from build123d import *

# Parameters (mm, degrees)
F0_W          = 80
F0_H          = 7
F0_R          = 2.6
F1_DEPTH      = 11.5
F2_R          = 3
F3_DEPTH      = 5
F4_R          = 3
F5_DEPTH      = 80.001
F6_W          = 4
F6_H          = 3.5
F7_DEPTH      = 39
F7_DEPTH_BACK = 39
F8_SIZE2      = 6.9282032303
F8_SIZE       = 4
F9_SIZE2      = 1.558836
F9_SIZE       = 0.89999
F10_W         = 2
F10_H         = 10.311042398
F11_DEPTH     = 80.001
F12_R         = 3.5
F13_DEPTH     = 1.75
F14_T4_DEPTH  = 17.5408905874
F14_T9_DEPTH  = 17.5408905874
F15_W         = 3
F15_H         = 1.3
F16_DEPTH     = 7.0010001


# Not quite as in the source:
# - a fillet or chamfer that OpenCascade refuses, or shapes differently, is made with other operations: its cross-section is extruded or revolved along the edge and cut away or added
# - a fillet or chamfer is up to 0.001 mm smaller than in the source, because OpenCascade refuses the exact size


with BuildPart() as f1:
    # F0 (on Front) → F1 (new body)
    with BuildSketch(Plane.XZ):
        Rectangle(F0_W, F0_H)
        with Locations((-33, 0)):
            Circle(F0_R, mode=Mode.SUBTRACT)
        with Locations((-22, 0)):
            Circle(F0_R, mode=Mode.SUBTRACT)
        with Locations((-11, 0)):
            Circle(F0_R, mode=Mode.SUBTRACT)
        Circle(F0_R, mode=Mode.SUBTRACT)
        with Locations((11, 0)):
            Circle(F0_R, mode=Mode.SUBTRACT)
        with Locations((22, 0)):
            Circle(F0_R, mode=Mode.SUBTRACT)
        with Locations((33, 0)):
            Circle(F0_R, mode=Mode.SUBTRACT)
    extrude(amount=F1_DEPTH)

    # F2 (on face) → F3 (cut)
    with BuildSketch(Plane(origin=(0, 0, 0), x_dir=(-1, 0, 0), z_dir=(0, 1, 0))):
        Circle(F2_R)
        with Locations((11, 0)):
            Circle(F2_R)
        with Locations((22, 0)):
            Circle(F2_R)
        with Locations((33, 0)):
            Circle(F2_R)
        with Locations((-11, 0)):
            Circle(F2_R)
        with Locations((-22, 0)):
            Circle(F2_R)
        with Locations((-33, 0)):
            Circle(F2_R)
    extrude(amount=-F3_DEPTH, mode=Mode.SUBTRACT)

    # F4 (on face) → F5 (cut, through all)
    with BuildSketch(Plane(origin=(-40, 0, 0), x_dir=(0, -1, 0), z_dir=(-1, 0, 0))):
        Circle(F4_R)
    extrude(amount=-F5_DEPTH, mode=Mode.SUBTRACT)

    # F6 (on Right) → F7 (cut, two sides)
    with BuildSketch(Plane.YZ) as f7_sk:
        with Locations((-3, 0)):
            Rectangle(F6_W, F6_H)
    extrude(amount=-F7_DEPTH, mode=Mode.SUBTRACT)
    extrude(f7_sk.sketch, amount=F7_DEPTH_BACK, mode=Mode.SUBTRACT)

    # F8
    f8_edges = [f1.edges().sort_by_distance(p)[0] for p in [
        (-40, -11.5, 0),
        (40, -11.5, 0),
    ]]
    f8_side = f1.faces().sort_by_distance((39.196943, -11.5, 0))[0]
    chamfer(f8_edges, length=F8_SIZE, length2=F8_SIZE2, reference=f8_side)

    # F9 (size 0.9 and 1.5588457268 in the source; OpenCascade refuses exactly that, so slightly less here)
    f9_edges = [f1.edges().sort_by_distance(p)[0] for p in [
        (0, -11.5, 3.5),
        (0, -11.5, -3.5),
    ]]
    f9_side = f1.faces().sort_by_distance((0, -11.5, 2.776605))[0]
    chamfer(f9_edges, length=F9_SIZE, length2=F9_SIZE2, reference=f9_side)

    # F10 (on face) → F11 (cut, through all)
    with BuildSketch(Plane(origin=(-40, 0, 0), x_dir=(0, -1, 0), z_dir=(-1, 0, 0))):
        Rectangle(F10_W, F10_H)
    extrude(amount=-F11_DEPTH, mode=Mode.SUBTRACT)

    # F12 (on face) → F13 (cut, through all)
    with BuildSketch(Plane(origin=(0, 0, -3.5), x_dir=(1, 0, 0), z_dir=(0, 0, -1))):
        with Locations((0, 1)):
            Circle(F12_R)
    extrude(amount=-F13_DEPTH, mode=Mode.SUBTRACT)

    # F14: fillet of radius 5 on 2 edges, made by hand


with BuildPart() as f14_tool2:
    # F14_s3 → F14_t4 (new body)
    with BuildSketch(Plane.XY.offset(5.6062317314)):
        with BuildLine():
            ThreePointArc((-6.8738635424, -1), (-4.60515051, -1.5443360566), (-2.8304143998, -3.0588235294))
            ThreePointArc((-2.8304143998, -3.0588235294), (-3.3283967912, -2.0824854735), (-3.5, -1))
            Line((-3.5, -1), (-6.8738635424, -1))
        make_face()
    extrude(amount=-F14_T4_DEPTH)

    split(bisect_by=Plane.XY.offset(1.75), keep=Keep.BOTTOM)


with BuildPart() as f1_1:
    add(f1.part)

    # F14_t1: cut F14_tool2
    add(f14_tool2.part, mode=Mode.SUBTRACT)


with BuildPart() as f14_tool7:
    # F14_s8 → F14_t9 (new body)
    with BuildSketch(Plane.XY.offset(-11.9346588561)):
        with BuildLine():
            ThreePointArc((2.8304143998, -3.0588235294), (4.60515051, -1.5443360566), (6.8738635424, -1))
            Line((6.8738635424, -1), (3.5, -1))
            ThreePointArc((3.5, -1), (3.3283967912, -2.0824854735), (2.8304143998, -3.0588235294))
        make_face()
    extrude(amount=F14_T9_DEPTH)

    split(bisect_by=Plane.XY.offset(1.75), keep=Keep.BOTTOM)


with BuildPart() as f1_2:
    add(f1_1.part)

    # F14_t6: cut F14_tool7
    add(f14_tool7.part, mode=Mode.SUBTRACT)

    # F15 (on face) → F16 (cut, through all)
    with BuildSketch(Plane.XY.offset(3.5)):
        with Locations((37.5, -4.35)):
            Rectangle(F15_W, F15_H)
        with Locations((16.5, -4.35)):
            Rectangle(F15_W, F15_H)
        with Locations((-16.5, -4.35)):
            Rectangle(F15_W, F15_H)
        with Locations((-37.5, -4.35)):
            Rectangle(F15_W, F15_H)
    extrude(amount=-F16_DEPTH, mode=Mode.SUBTRACT)


solid = f1_2.part
Design review of the part built by this model. Coordinates are the model's own, in mm. A direction names the side the tool comes from. Coordinates: 2 decimals unless noted, no trailing zeros. Order: outer loops, then holes, each group sorted by start corner. A loop starts at its lowest first (then second) coordinate and runs counter-clockwise, first axis right, second up.
Item 1: Take a section at C-C, the plane y = -6.5. Write out the cut boundary in (x, z), then the cut area to 3 significant figures.
Item 2: The part is to be moulded in two halves that separate along Z. For faces 1 (the cylindrical face through (-19.52, -8.2, 0.78)), 2 (the flat face through (18, -4, 3)), say which applies: pulls with the +Z half, pulls with the -Z half, needs draft (parallel to the pull), parting line crosses it, or undercut.
Item 3: For line 1 (Z direction, x = 33, y = -7.25); line 2 (Z direction, x = -1, y = -2); line 3 (Y direction, x = 17.5, z = 0.75), list the stretches that pass through material, from the lowest coordinate up.
Item 4: Take a section at B-B, the plane x = -26. Write out the cut boundary in (y, z), then the cut area to 3 significant figures.
Item 5: For faces 3 (the cylindrical face through (-11, -3, 3)), 4 (the flat face through (-17, -3.7, -3)), 5 (the flat face through (39, -4, 0)), list the 3-axis set-ups (+Z, -Z, +X, -X, +Y, -Y) from which the entire face can be reached by the end or side of a thin tool; tool diameter is ignored.
Item 6: For pin 1 Ø2 at (y, z) = (-7.5, 2) entering from -X; pin 2 Ø0.9 at (x, z) = (-38, -3) entering from -Y, all flat-tipped, find the tip position at first contact; note any pin that passes through.
The answers:
1. outline: (-38.89, -3.5) - (38.89, -3.5) - (38.89, 3.5) - (-38.89, 3.5) - close; hole circle Ø5.2 at (-33, 0); hole circle Ø5.2 at (-22, 0); hole circle Ø5.2 at (-11, 0); hole circle Ø5.2 at (0, 0); hole circle Ø5.2 at (11, 0); hole circle Ø5.2 at (22, 0); hole circle Ø5.2 at (33, 0)
1. area: 396 mm2
2. face 1: undercut
2. face 2: needs draft
3. line 1: z = -3.5 to -2.6, 2.6 to 3.5
3. line 2: z = 2.83 to 3.5
3. line 3: y = -11.5 to -5
4. outline: (-11.5, -2.6) - (-9.94, -3.5) - (-1, -3.5) - (-1, -2.83) arc R3 cw to (-2.44, -1.75) - (-5, -1.75) - (-5, 1.75) - (-2.44, 1.75) arc R3 cw to (-1, 2.83) - (-1, 3.5) - (-9.94, 3.5) - (-11.5, 2.6) - close
4. area: 56.2 mm2
5. face 3: +Y
5. face 4: +Z, -Z
5. face 5: none
6. pin 1: stops at x = -38.89
6. pin 2: stops at y = -8.82
